from build123d import *

# Parameters (mm, degrees)
SKETCH1_W           = 218.9
SKETCH1_H           = 66.5
SKETCH1_R           = 2.25
SKETCH1_W_2         = 4
SKETCH1_H_2         = 45
BOSS_EXTRUDE1_DEPTH = 1.6
FILLET1_R           = 1
SKETCH3_W           = 4
SKETCH3_H           = 2.831639971
BOSS_EXTRUDE2_DEPTH = 5.1


with BuildPart() as part:
    # Sketch1 → Boss-Extrude1 (new body)
    with BuildSketch(Plane(origin=(0, 0, 0), x_dir=(1, 0, 0), z_dir=(0, 1, 0))):
        with Locations((109.45, 33.25)):
            Rectangle(SKETCH1_W, SKETCH1_H)
        with Locations((11, 63)):
            Circle(SKETCH1_R, mode=Mode.SUBTRACT)
        with Locations((63.4, 63)):
            Circle(SKETCH1_R, mode=Mode.SUBTRACT)
        with Locations((145.9, 63)):
            Circle(SKETCH1_R, mode=Mode.SUBTRACT)
        with Locations((207.9, 63)):
            Circle(SKETCH1_R, mode=Mode.SUBTRACT)
        with Locations((5.75, 5)):
            Circle(SKETCH1_R, mode=Mode.SUBTRACT)
        with Locations((109.45, 4.3)):
            Circle(SKETCH1_R, mode=Mode.SUBTRACT)
        with Locations((213.15, 5)):
            Circle(SKETCH1_R, mode=Mode.SUBTRACT)
        with Locations((22, 35)):
            Rectangle(SKETCH1_W_2, SKETCH1_H_2, mode=Mode.SUBTRACT)
        with Locations((49.5, 35)):
            Rectangle(SKETCH1_W_2, SKETCH1_H_2, mode=Mode.SUBTRACT)
        with Locations((77, 35)):
            Rectangle(SKETCH1_W_2, SKETCH1_H_2, mode=Mode.SUBTRACT)
        with Locations((104.5, 35)):
            Rectangle(SKETCH1_W_2, SKETCH1_H_2, mode=Mode.SUBTRACT)
        with Locations((132, 35)):
            Rectangle(SKETCH1_W_2, SKETCH1_H_2, mode=Mode.SUBTRACT)
        with Locations((159.5, 35)):
            Rectangle(SKETCH1_W_2, SKETCH1_H_2, mode=Mode.SUBTRACT)
        with Locations((187, 35)):
            Rectangle(SKETCH1_W_2, SKETCH1_H_2, mode=Mode.SUBTRACT)
        with Locations((214.5, 35)):
            Rectangle(SKETCH1_W_2, SKETCH1_H_2, mode=Mode.SUBTRACT)
    extrude(amount=BOSS_EXTRUDE1_DEPTH)

    # Fillet1
    fillet1_edges = [part.edges().sort_by_distance(p)[0] for p in [
        (0, 0.8, -66.5),
        (218.9, 0.8, -66.5),
        (218.9, 0.8, 0),
        (0, 0.8, 0),
    ]]
    fillet(fillet1_edges, radius=FILLET1_R)

    # Sketch3 → Boss-Extrude2 (add)
    with BuildSketch(Plane(origin=(0, 0, 0), x_dir=(1, 0, 0), z_dir=(0, 1, 0))):
        with Locations((22, 58.915819986)):
            Rectangle(SKETCH3_W, SKETCH3_H)
    extrude(amount=BOSS_EXTRUDE2_DEPTH)


solid = part.part
Build history of the part. All positions in model axes, mm. Give positions to 0.01 mm unless a question says otherwise; leave off trailing zeros. Order: outer loops, then holes, each group sorted by start corner. A loop starts at its lowest first (then second) coordinate and runs counter-clockwise, first axis right, second up. Notation, with made-up numbers: M 9.25,-37.75 L 54.25,-37.75 A33 cw 54.25,-1.75 Z; hole C 55,56.5 d1. An arc over 180 degrees is marked long. Use one line per item in the form item = value.
1) Probe probe 1 along X at (y, z) = (0.45, -63); probe 2 along Z at (x, y) = (213.15, 0.55); probe 3 along Z at (x, y) = (11, 0.7). List the from-to ranges inside material, lowest first.
Calculated:
probe_1 = 0 to 8.75, 13.25 to 61.15, 65.65 to 143.65, 148.15 to 205.65, 210.15 to 218.9
probe_2 = -66.5 to -57.5, -12.5 to -7.25, -2.75 to 0
probe_3 = -66.5 to -65.25, -60.75 to 0
2) Saw through at B-B (z = -18). State how many separate pieces and enclosed holes the cut face has, plus the area to 3 significant figures.
Calculated:
separate_pieces = 9
enclosed_holes = 0
area = 299 mm2
3) Saw through at A-A (x = 5.75). Give the cut face in (y, z), plus the area to 3 significant figures.
Calculated:
outline = M 0,-66.5 L 1.6,-66.5 L 1.6,-7.25 L 0,-7.25 Z; M 0,-2.75 L 1.6,-2.75 L 1.6,0 L 0,0 Z
area = 99.2 mm2
4) Saw through at D-D (x = 119.5). Give the cut face in (y, z).
Calculated:
outline = M 0,-66.5 L 1.6,-66.5 L 1.6,0 L 0,0 Z
5) Drop flat-ended pins along their axis: pin 1 (6 mm diameter, centred on x = 109, z = -58, fed in from -Y); pin 2 (6 mm diameter, centred on x = 11, z = -63, fed in from +Y); pin 3 (4 mm diameter, centred on x = 207.9, z = -63, fed in from -Y). Give the stop position or say it passes through.
Calculated:
pin_1 = 0
pin_2 = 1.6
pin_3 = through
6) Saw through at C-C (y = 4.25). Give the cut face in (x, z).
Calculated:
outline = M 20,-60.33 L 24,-60.33 L 24,-57.5 L 20,-57.5 Z
7) Two-plate mould, pull along Z, no slides. Class faces 1 (the face through (22, 3, -60.332)), 2 (the face through (108, 0, -34)), 3 (the face through (215.296, 0.789, -5.676)): released by +Z, released by -Z, zero draft, split by the parting line, or undercut.
Calculated:
face_1 = released by -Z
face_2 = zero draft
face_3 = undercut
